```python
from build123d import *

# Parameters (mm, degrees)
F1_DEPTH = 76.2


with BuildPart() as f1:
    # F0 (on Right) → F1 (new body)
    with BuildSketch(Plane.YZ):
        Polygon((-82.55, 66.675), (-82.55, 3.175), (-76.2, 3.175), (-76.2, 60.195141), (-76.2, 66.675), align=None)
        Polygon((-76.2, 3.175), (-82.55, 3.175), (-82.55, -3.175), (82.55, -3.175), (82.55, 3.175), (70.252687, 3.175), (-23.647007, 3.175), (-31.397808, 3.175), align=None)
        Polygon((-76.2, 66.675), (-76.2, 60.195141), (-31.397808, 42.751778), (-23.647007, 39.734068), (70.252687, 3.175), (82.55, 3.175), align=None)
        Polygon((-31.397808, 42.751778), (-31.397808, 3.175), (-23.647007, 3.175), (-23.647007, 39.734068), align=None)
    extrude(amount=-F1_DEPTH)


solid = f1.part
```
Model file for the job. Use its own axes, mm. A direction names the side the tool comes from. Round coordinates to 2 decimals unless told otherwise and drop trailing zeros. Order: outer loops, then holes, each group sorted by start corner. A loop starts at its lowest first (then second) coordinate and runs counter-clockwise, first axis right, second up. Notation, with made-up numbers: M -23,28.5 L 18,28.5 A24 cw 18,42.5 Z; hole C 89.25,-5 d3. An arc over 180 degrees is marked long. Use CSV: the item, a comma, the result in double quotes.
Item 1: Pin check, flat tips, straight feed: pin 1 (22.5 mm diameter, centred on x = -42, y = -44.5, fed in from +Z) (3 decimals); pin 2 (12 mm diameter, centred on y = -62.5, z = 52, fed in from +X); pin 3 (2 mm diameter, centred on x = -28.5, z = 32, fed in from +Y); pin 4 (23 mm diameter, centred on x = -44.5, y = 28, fed in from +Z) (3 decimals). Stop position of each tip, or through.
Worked answers:
pin 1,"z = 58.495"
pin 2,"x = 0"
pin 3,"y = 12.99"
pin 4,"z = 29.595"
Item 2: Probe probe 1 along Z at (x, y) = (-62.5, 28.5) (3 decimals); probe 2 along Z at (x, y) = (-63, -47.5) (3 decimals); probe 3 along Z at (x, y) = (-49.5, 73.5) (3 decimals). List the from-to ranges inside material, lowest first.
Worked answers:
probe 1,"-3.175 to 3.175, 19.431 to 24.795"
probe 2,"-3.175 to 3.175, 49.021 to 55.195"
probe 3,"-3.175 to 6.795"
Item 3: Saw through at C-C (z = 15). List the corners of the cut face in (x, y).
Worked answers:
outline,"M -76.2,-82.55 L 0,-82.55 L 0,-76.2 L -76.2,-76.2 Z; M -76.2,-31.4 L 0,-31.4 L 0,-23.65 L -76.2,-23.65 Z; M -76.2,39.88 L 0,39.88 L 0,52.99 L -76.2,52.99 Z"
Item 4: Saw through at D-D (z = 52). List the corners of the cut face in (x, y).
Worked answers:
outline,"M -76.2,-82.55 L 0,-82.55 L 0,-76.2 L -76.2,-76.2 Z; M -76.2,-55.15 L 0,-55.15 L 0,-39.51 L -76.2,-39.51 Z"
Item 5: Saw through at B-B (y = -70). List the corners of the cut face in (x, z) (3 decimals), plus the area to 3 significant figures.
Worked answers:
outline,"M -76.2,-3.175 L 0,-3.175 L 0,3.175 L -76.2,3.175 Z; M -76.2,57.781 L 0,57.781 L 0,64.195 L -76.2,64.195 Z"
area,"973 mm²"
Item 6: Which spindle directions (+Z, -Z, +X, -X, +Y, -Y) get a long thin tool onto all of the face, cutting with end or side? Do faces 4 (the face through (-37.57, 4.29, 34.48)), 5 (the face through (-38, -53, 3.175)). Say none if no direction does.
Worked answers:
face 4,"+Z, +X, -X, +Y"
face 5,"+X, -X"
Item 7: Saw through at A-A (x = -14). List the corners of the cut face in (y, z) (3 decimals), plus the area to 3 significant figures.
Worked answers:
outline,"M -82.55,-3.175 L 82.55,-3.175 L 82.55,3.175 L -76.2,66.675 L -82.55,66.675 Z; hole M -76.2,3.175 L -31.398,3.175 L -31.398,42.752 L -76.2,60.195 Z; hole M -23.647,3.175 L 70.253,3.175 L -23.647,39.734 Z"
area,"2,610 mm²"
Item 8: Pull direction Z, two halves, no side cores. Call faces 1 (the face through (-38, 82.55, 0)), 2 (the face through (-37.57, 22.65, 21.71)), 3 (the face through (-38, -1, -3.175)): released by +Z, released by -Z, zero draft, split by the parting line, or undercut.
Worked answers:
face 1,"zero draft"
face 2,"undercut"
face 3,"released by -Z"
